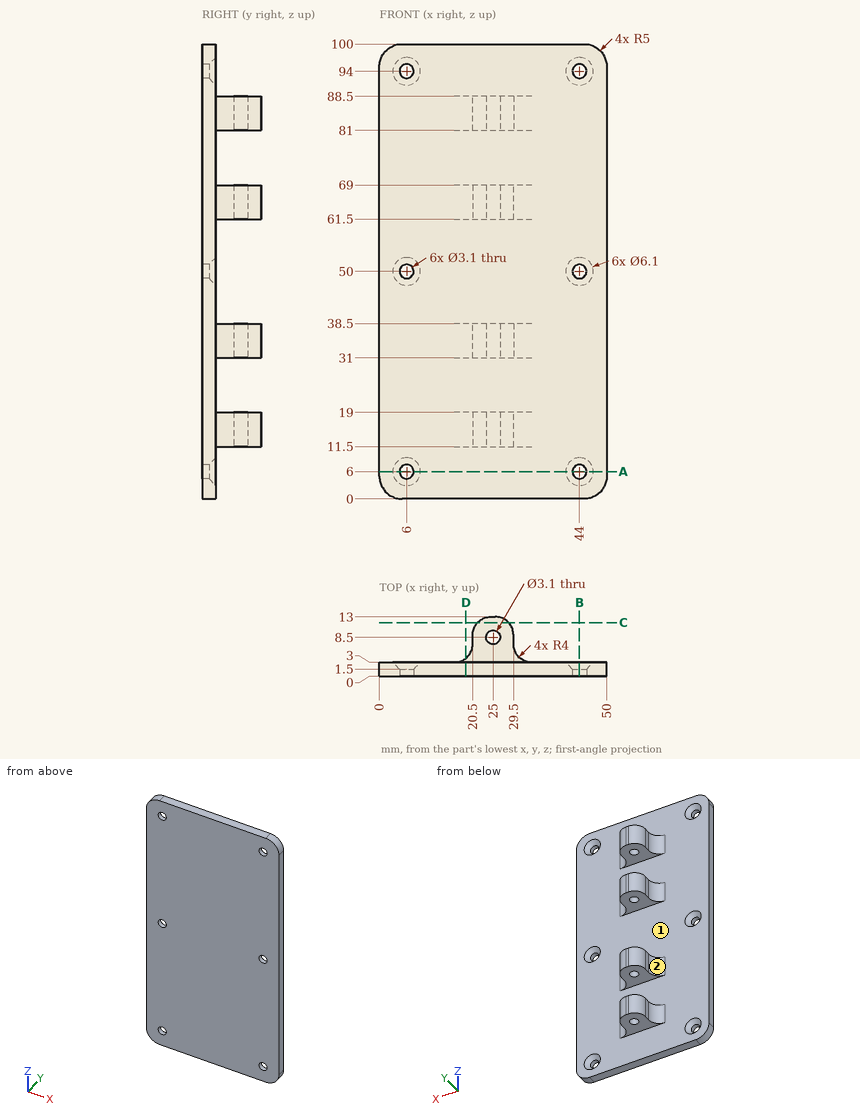
Job drawing, mm, ordinate dimensions from the low corner. One solid piece. A direction names the side the tool comes from. Coordinates: 2 decimals unless noted, no trailing zeros. Write each loop counter-clockwise with the first axis right and the second up, starting at its lowest first coordinate (ties: lowest second). Pieces come first, ordered by that corner, then holes.
Item 1: Which spindle directions (+Z, -Z, +X, -X, +Y, -Y) get a long thin tool onto all of the face, cutting with end or side? Do the marked faces 1 and 2. Say none if no direction does.
Item 2: Slice it at C-C (y = 11.75). Write the cut outline in (x, z), and give its area (3 significant figures).
Item 3: Probe line 1 (Z direction, x = 44, y = 0.55); line 2 (X direction, y = 0.85, z = 50); line 3 (Z direction, x = 21, y = 8.75). List the from-to ranges inside material, lowest first.
Item 4: Pin check, flat tips, straight feed: pin 1 (0.6 mm diameter, centred on y = 7.5, z = 84, fed in from -X); pin 2 (4 mm diameter, centred on x = 6, z = 94, fed in from -Y); pin 3 (4 mm diameter, centred on x = 25, y = 8.5, fed in from -Z); pin 4 (4 mm diameter, centred on x = 25, y = 8.5, fed in from +Z). Stop position of each tip, or through.
Item 5: Slice it at B-B (x = 44). Write the cut outline in (y, z).
Item 6: Slice it at D-D (x = 19). Write the cut outline in (y, z).
Item 7: Slice it at A-A (z = 6). Write the cut outline in (x, y), and give its area (3 significant figures).
Results found:
1. face 1: +Y
1. face 2: +Z, -Z, -X, +Y
2. outline: (21.6, 11.5) - (28.4, 11.5) - (28.4, 19) - (21.6, 19) - close; (21.6, 31) - (28.4, 31) - (28.4, 38.5) - (21.6, 38.5) - close; (21.6, 61.5) - (28.4, 61.5) - (28.4, 69) - (21.6, 69) - close; (21.6, 81) - (28.4, 81) - (28.4, 88.5) - (21.6, 88.5) - close
2. area: 204 mm2
3. line 1: z = 0 to 4.45, 7.55 to 48.45, 51.55 to 92.45, 95.55 to 100
3. line 2: x = 0 to 4.45, 7.55 to 42.45, 45.55 to 50
3. line 3: z = 11.5 to 19, 31 to 38.5, 61.5 to 69, 81 to 88.5
4. pin 1: stops at x = 20.5
4. pin 2: stops at y = 0
4. pin 3: stops at z = 11.5
4. pin 4: stops at z = 88.5
5. outline: (0, 0) - (3, 0) - (3, 2.95) - (1.5, 4.45) - (0, 4.45) - close; (0, 7.55) - (1.5, 7.55) - (3, 9.05) - (3, 46.95) - (1.5, 48.45) - (0, 48.45) - close; (0, 51.55) - (1.5, 51.55) - (3, 53.05) - (3, 90.95) - (1.5, 92.45) - (0, 92.45) - close; (0, 95.55) - (1.5, 95.55) - (3, 97.05) - (3, 100) - (0, 100) - close
6. outline: (0, 0) - (3, 0) - (3, 11.5) - (3.88, 11.5) - (3.88, 19) - (3, 19) - (3, 31) - (3.88, 31) - (3.88, 38.5) - (3, 38.5) - (3, 61.5) - (3.88, 61.5) - (3.88, 69) - (3, 69) - (3, 81) - (3.88, 81) - (3.88, 88.5) - (3, 88.5) - (3, 100) - (0, 100) - close
7. outline: (0, 0) - (4.45, 0) - (4.45, 1.5) - (2.95, 3) - (0, 3) - close; (7.55, 0) - (42.45, 0) - (42.45, 1.5) - (40.95, 3) - (9.05, 3) - (7.55, 1.5) - close; (45.55, 0) - (50, 0) - (50, 3) - (47.05, 3) - (45.55, 1.5) - close
7. area: 127 mm2
